Design review of the part built by this model. Coordinates are the model's own, in mm. Face numbers are marked on the shaded views. A direction names the side the tool comes from. Round coordinates to 2 decimals unless told otherwise and drop trailing zeros. Loops run counter-clockwise (first coordinate to the right, second up) from the corner with the lowest first, then second, coordinate; pieces in that order, holes last. Notation, with made-up numbers: (81.5, 65.25) - (101.5, 65.25) arc R10 cw to (101.5, 73.25) - close; hole circle Ø7 at (25.25, 80). An arc over 180 degrees is marked (long way). Answer as CSV lines item,"result". Start each with the question number.
(1) Wall thickness on L1, parallel to Z at x = 27, y = -10.5; L2, parallel to Z at x = 28, y = -8.25; L3, parallel to Y at x = 52, z = 32: over which ranges is each line inside the solid? List them lowest first.
(2) Consider section B-B (z = 49). Give the boundary of the cut face in (x, y).
(3) Consider section A-A (x = 107). Give the boundary of the cut face in (y, z).
(4) For the marked faces 5, 6 and 7, list the 3-axis set-ups (+Z, -Z, +X, -X, +Y, -Y) from which the entire face can be reached by the end or side of a thin tool; tool diameter is ignored.
(5) Mouldability with a two-part tool opening along X and no side actions: class the marked faces 1, 2, 3 and 4 as released by +X, released by -X, zero draft, split by the parting line, or undercut.
(6) For P1, Ø5, axis at x = 87, y = -13, coming from the +Z side; P2, Ø11, axis at x = 117.5, z = 7, coming from the -Y side; P3, Ø0.6, axis at y = -1.5, z = 4, coming from the +X side; P4, Ø10, axis at x = 110.5, z = 17.5, coming from the -Y side, all flat-tipped, find the tip position at first contact; note any pin that passes through.
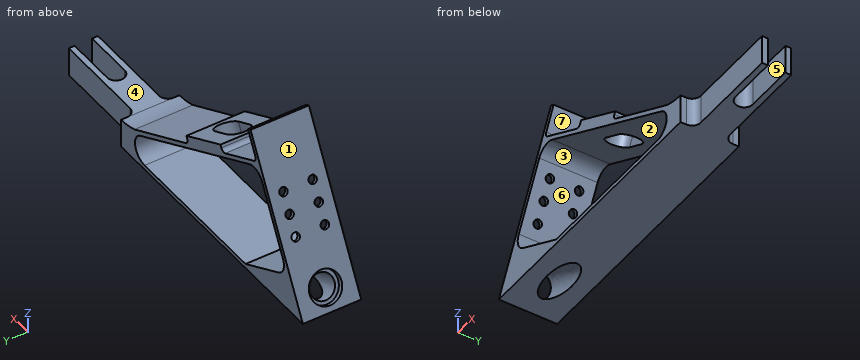
from build123d import *

# Parameters (mm, degrees)
F1_DEPTH  = 20
F2_R      = 1.5
F3_W      = 35
F3_H      = 5
F4_DEPTH  = 10.001
F5_R      = 3
F7_DEPTH  = 10.001
F9_DEPTH  = 4
F11_DEPTH = 20.001
F12_R     = 5.5
F12_R_2   = 4.25
F13_DEPTH = 2
F14_DEPTH = 115.7145863741
F15_R     = 1.395
F16_DEPTH = 25


with BuildPart() as f1:
    # F0 (on Front) → F1 (new body)
    with BuildSketch(Plane.XZ):
        with BuildLine():
            Line((27.3453882208, 53.4062706342), (0, 0))
            Line((0, 0), (130, 0))
            Line((130, 0), (130, 10))
            Line((130, 10), (95, 10))
            ThreePointArc((95, 10), (91.4222885738, 10.322602282), (87.9599949346, 11.2800019049))
            Line((87.9599949346, 11.2800019049), (59.727160706, 25.5913320091))
            Line((59.727160706, 25.5913320091), (60.8665518818, 27.8165932856))
            Line((60.8665518818, 27.8165932856), (43.0644616704, 36.9317226925))
            Line((43.0644616704, 36.9317226925), (41.9250704946, 34.7064614161))
            Line((41.9250704946, 34.7064614161), (24.1229802832, 43.821590823))
            Line((24.1229802832, 43.821590823), (28.6805449866, 52.7226359287))
            Line((28.6805449866, 52.7226359287), (27.3453882208, 53.4062706342))
        make_face()
    extrude(amount=F1_DEPTH)

    # F2
    f2_edges = [f1.edges().sort_by_distance(p)[0] for p in [
        (59.727161, -10, 25.591332),
        (24.12298, -10, 43.821591),
        (41.92507, -10, 34.706461),
    ]]
    fillet(f2_edges, radius=F2_R)

    # F3 (on face) → F4 (cut, through all)
    with BuildSketch(Plane.XY.offset(10)):
        with Locations((112.5, -2.5)):
            Rectangle(F3_W, F3_H)
        with Locations((112.5, -17.5)):
            Rectangle(F3_W, F3_H)
    extrude(amount=-F4_DEPTH, mode=Mode.SUBTRACT)

    # F5
    f5_edges = [f1.edges().sort_by_distance(p)[0] for p in [
        (95, -15, 5),
        (95, -5, 5),
    ]]
    fillet(f5_edges, radius=F5_R)

    # F6 (on face) → F7 (cut, through all)
    with BuildSketch(Plane.XY.offset(10)):
        with BuildLine():
            Line((130, -13), (130, -7))
            Line((130, -7), (113, -7))
            ThreePointArc((113, -7), (110, -10), (113, -13))
            Line((113, -13), (130, -13))
        make_face()
    extrude(amount=-F7_DEPTH, mode=Mode.SUBTRACT)

    # F8 (on face) → F9 (cut)
    with BuildSketch(Plane(origin=(23.9272146932, 0, 46.7304868049), x_dir=(0.8901045106, 0, -0.4557564703), z_dir=(0.4557564703, 0, 0.8901045106))):
        with BuildLine():
            Line((35, -6), (28, -6))
            ThreePointArc((28, -6), (24, -10), (28, -14))
            Line((28, -14), (35, -14))
            ThreePointArc((35, -14), (39, -10), (35, -6))
        make_face()
    extrude(amount=-F9_DEPTH, mode=Mode.SUBTRACT)

    # F10 (on face) → F11 (cut, through all)
    with BuildSketch(Plane.XZ.offset(20)):
        with BuildLine():
            ThreePointArc((27.8898681305, 40.2076517054), (24.0754335556, 40.5154662833), (21.1605632259, 38.0359115043))
            Line((21.1605632259, 38.0359115043), (10.4502861728, 17.1184555059))
            ThreePointArc((10.4502861728, 17.1184555059), (10.1424715949, 13.304020931), (12.6220263739, 10.3891506013))
            Line((12.6220263739, 10.3891506013), (29.9827739665, 1.5))
            Line((29.9827739665, 1.5), (82.7510373087, 1.5))
            ThreePointArc((82.7510373087, 1.5), (87.6117272167, 5.3279532356), (85.0298196604, 10.9505225529))
            Line((85.0298196604, 10.9505225529), (27.8898681305, 40.2076517054))
        make_face()
    extrude(amount=-F11_DEPTH, mode=Mode.SUBTRACT)

    # F12 (on face) → F13 (cut)
    with BuildSketch(Plane(origin=(0, 0, 0), x_dir=(0, -1, 0), z_dir=(-0.8901045106, 0, 0.4557564703))):
        with Locations((10, 7.5)):
            Circle(F12_R)
        with Locations((10, 7.5)):
            Circle(F12_R_2, mode=Mode.SUBTRACT)
    extrude(amount=-F13_DEPTH, mode=Mode.SUBTRACT)

    # F14 (cut, through all): a face of the model
    f14_faces = [f1.faces().sort_by_distance(p)[0] for p in [
        (3.4181735276, -10, 6.6757838293),
    ]]
    extrude(f14_faces, amount=-F14_DEPTH, mode=Mode.SUBTRACT)

    # F15 (on face) → F16 (cut)
    with BuildSketch(Plane(origin=(0, 0, 0), x_dir=(0, -1, 0), z_dir=(-0.8901045106, 0, 0.4557564703))):
        with Locations((5, 25)):
            Circle(F15_R)
        with Locations((5, 39)):
            Circle(F15_R)
        with Locations((5, 32)):
            Circle(F15_R)
        with Locations((15, 39)):
            Circle(F15_R)
        with Locations((15, 32)):
            Circle(F15_R)
        with Locations((15, 25)):
            Circle(F15_R)
    extrude(amount=-F16_DEPTH, mode=Mode.SUBTRACT)


solid = f1.part
Determined:
1,L1,"z = 0 to 3.03, 40.56 to 42.35, 49.44 to 52.73"
1,L2,"z = 0 to 2.52, 40.15 to 41.84, 51.39 to 53.07"
1,L3,"y = -20 to -14, -6 to 0"
2,outline,"(25.09, -20) - (26.77, -20) - (26.77, 0) - (25.09, 0) - close"
3,outline,"(-15, 0) - (-5, 0) - (-5, 10) - (-15, 10) - close"
4,face 5,"+Z, -Z, +X"
4,face 6,"+Y, -Y"
4,face 7,"+X, +Y, -Y"
5,face 1,"released by -X"
5,face 2,"undercut"
5,face 3,"undercut"
5,face 4,"zero draft"
6,P1,"stops at z = 13.03"
6,P2,"stops at y = -15"
6,P3,"stops at x = 95"
6,P4,"passes through"
